Geometry check sheet. Reference: drawing and pictorial views, mm from the part's lowest x, y, z. Round coordinates to 2 decimals unless told otherwise and drop trailing zeros. Order: outer loops, then holes, each group sorted by start corner. A loop starts at its lowest first (then second) coordinate and runs counter-clockwise, first axis right, second up.
(1) Sectioned sample at C-C, the plane x = 33. Enter the section's corners in (y, z) (1 decimal), and give its area (3 significant figures).
(2) Sectioned sample at B-B, the plane y = 3.25. Enter the section's corners in (x, z) (1 decimal), and give its area (3 significant figures).
(3) Mould release check, pull along Z, two halves, no side actions. Record for the marked faces 1, 2 and 3: released by +Z, released by -Z, zero draft, split by the parting line, or undercut.
(4) Thickness scan on probe 1 along Z at (x, y) = (35, 4) (1 decimal); probe 2 along Y at (x, z) = (35, 10); probe 3 along Z at (x, y) = (34, 7.5) (1 decimal). Record the ranges inside material, lowest first.
(5) Sectioned sample at A-A, the plane x = 28.5. Enter the section's corners in (y, z) (1 decimal).
(6) Sectioned sample at D-D, the plane y = 6. Enter the section's corners in (x, z) (1 decimal), and give its area (3 significant figures).
(7) Depth check by flat-ended pin: pin 1 (1.5 mm diameter, centred on x = 15, z = 11.5, fed in from +Y); pin 2 (1.5 mm diameter, centred on y = 4.5, z = 4, fed in from -X); pin 3 (12 mm diameter, centred on x = 18, z = 8.5, fed in from +Y). Enter the tip coordinate at first touch or a pass-through.
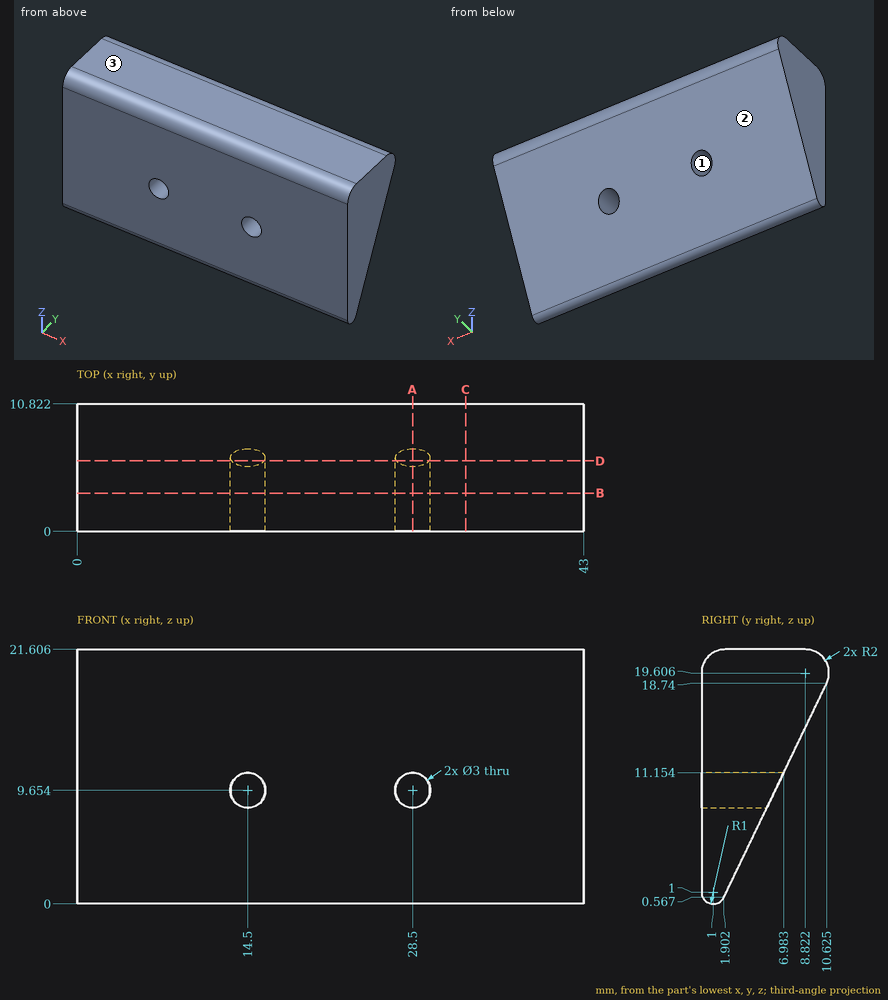
Derived:
1. outline: (0, 1) arc R1 ccw to (1.9, 0.6) - (10.6, 18.7) arc R2 ccw to (8.8, 21.6) - (2, 21.6) arc R2 ccw to (0, 19.6) - close
1. area: 144 mm2
2. outline: (0, 3.4) - (43, 3.4) - (43, 21.6) - (0, 21.6) - close; hole circle Ø3 at (14.5, 9.7); hole circle Ø3 at (28.5, 9.7)
2. area: 770 mm2
3. face 1: undercut
3. face 2: released by -Z
3. face 3: released by +Z
4. probe 1: z = 4.9 to 21.6
4. probe 2: y = 0 to 6.43
4. probe 3: z = 12.2 to 21.6
5. outline: (0, 1) arc R1 ccw to (1.9, 0.6) - (5.5, 8.2) - (0, 8.2) - close; (0, 11.2) - (7, 11.2) - (10.6, 18.7) arc R2 ccw to (8.8, 21.6) - (2, 21.6) arc R2 ccw to (0, 19.6) - close
6. outline: (0, 9.1) - (13.1, 9.1) arc R1.5 cw (long way) to (15.9, 9.1) - (27.1, 9.1) arc R1.5 cw (long way) to (29.9, 9.1) - (43, 9.1) - (43, 21.6) - (0, 21.6) - close
6. area: 527 mm2
7. pin 1: stops at y = 7.51
7. pin 2: passes through
7. pin 3: stops at y = 8.59
